Verification items for this drawing (mm, ordinates from the low corner). A direction names the side the tool comes from. Coordinates: 2 decimals unless noted, no trailing zeros. Write each loop counter-clockwise with the first axis right and the second up, starting at its lowest first coordinate (ties: lowest second). Pieces come first, ordered by that corner, then holes. Notation, with made-up numbers: M 24,17.5 L 65,17.5 A7 ccw 65,24.5 Z; hole C 85,35.5 d6. An arc over 180 degrees is marked long. Put each result on its own line as item: value. Start each with the question number.
1) Scan lines: line 1 along Y through (x, z) = (8.75, 7) (1 decimal); line 2 along Z through (x, y) = (12, 5.75). Record each from-to range of solid material in increasing order.
2) Set-up check for the marked faces 4 and 5: record each of +Z, -Z, +X, -X, +Y, -Y from which the full face is reachable in a straight line by a thin tool's end or side.
3) Gauge pin test, flat ends, axial feed: pin 1 (4 mm diameter, centred on x = 13, z = 14.5, fed in from -Y); pin 2 (5 mm diameter, centred on x = 10, y = 15, fed in from +Z). Record the tip position at first contact, or that the pin passes through.
4) Cross-section at B-B on x = 8.5. Record the cut outline in (y, z) (1 decimal).
5) Cross-section at A-A on y = 15.24. Record the cut outline in (x, z).
6) Mould release check, pull along Z, two halves, no side actions. Record for the marked faces 1, 2 and 3: released by +Z, released by -Z, zero draft, split by the parting line, or undercut.
7) Cross-section at D-D on x = 6.5. Record the cut outline in (y, z) (1 decimal), plus the area to 3 significant figures.
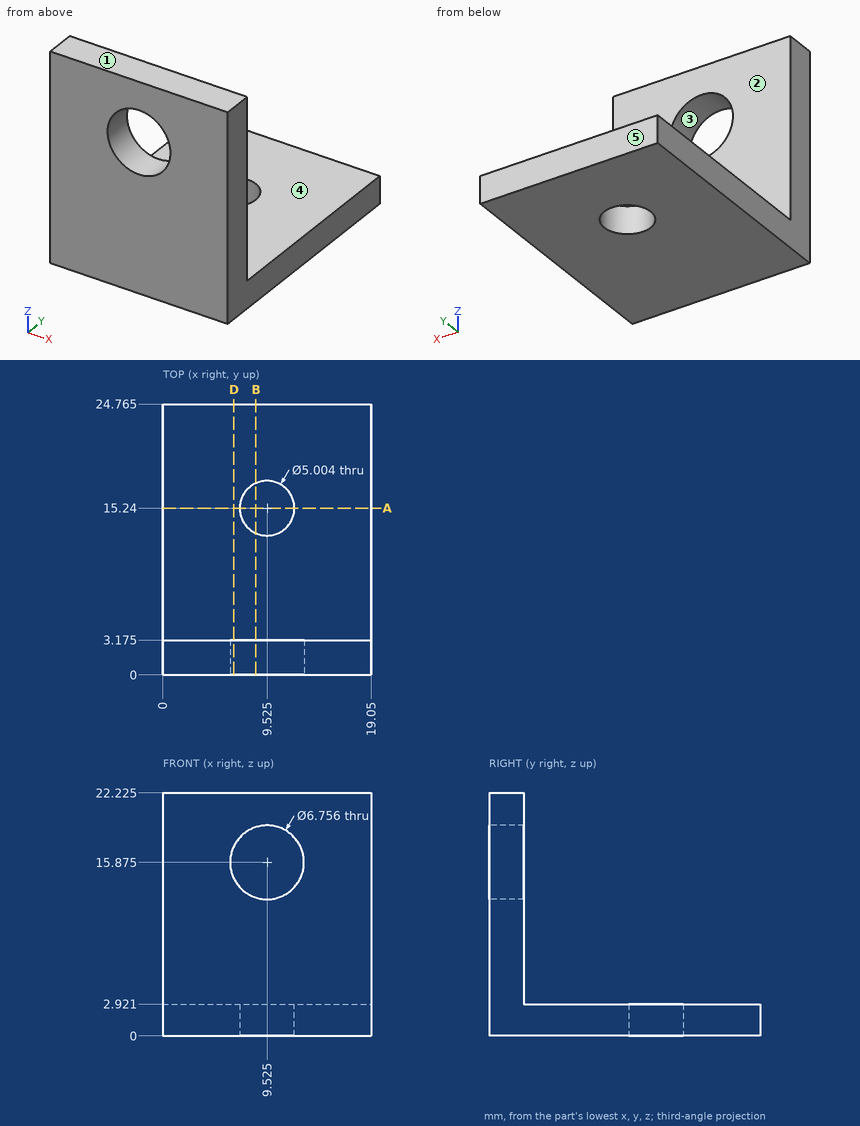
Answer key:
1. line 1: y = 0 to 3.2
1. line 2: z = 0 to 2.92
2. face 4: +Z, +X, -X, +Y
2. face 5: +Z, -Z, +X, -X, +Y
3. pin 1: stops at y = 0
3. pin 2: stops at z = 2.92
4. outline: M 0,0 L 13,0 L 13,2.9 L 3.2,2.9 L 3.2,12.7 L 0,12.7 Z; M 0,19.1 L 3.2,19.1 L 3.2,22.2 L 0,22.2 Z; M 17.5,0 L 24.8,0 L 24.8,2.9 L 17.5,2.9 Z
5. outline: M 0,0 L 7.02,0 L 7.02,2.92 L 0,2.92 Z; M 12.03,0 L 19.05,0 L 19.05,2.92 L 12.03,2.92 Z
6. face 1: released by +Z
6. face 2: zero draft
6. face 3: undercut
7. outline: M 0,0 L 24.8,0 L 24.8,2.9 L 3.2,2.9 L 3.2,14.4 L 0,14.4 Z; M 0,17.4 L 3.2,17.4 L 3.2,22.2 L 0,22.2 Z
7. area: 124 mm²
